Verification items for this drawing (mm, ordinates from the low corner). A direction names the side the tool comes from. Round coordinates to 2 decimals unless told otherwise and drop trailing zeros. Loops run counter-clockwise (first coordinate to the right, second up) from the corner with the lowest first, then second, coordinate; pieces in that order, holes last. Notation, with made-up numbers: M 24,18 L 58,18 A21 cw 58,56 Z; hole C 18,56.25 d3. An arc over 180 degrees is marked long. One line per item, written item: value.
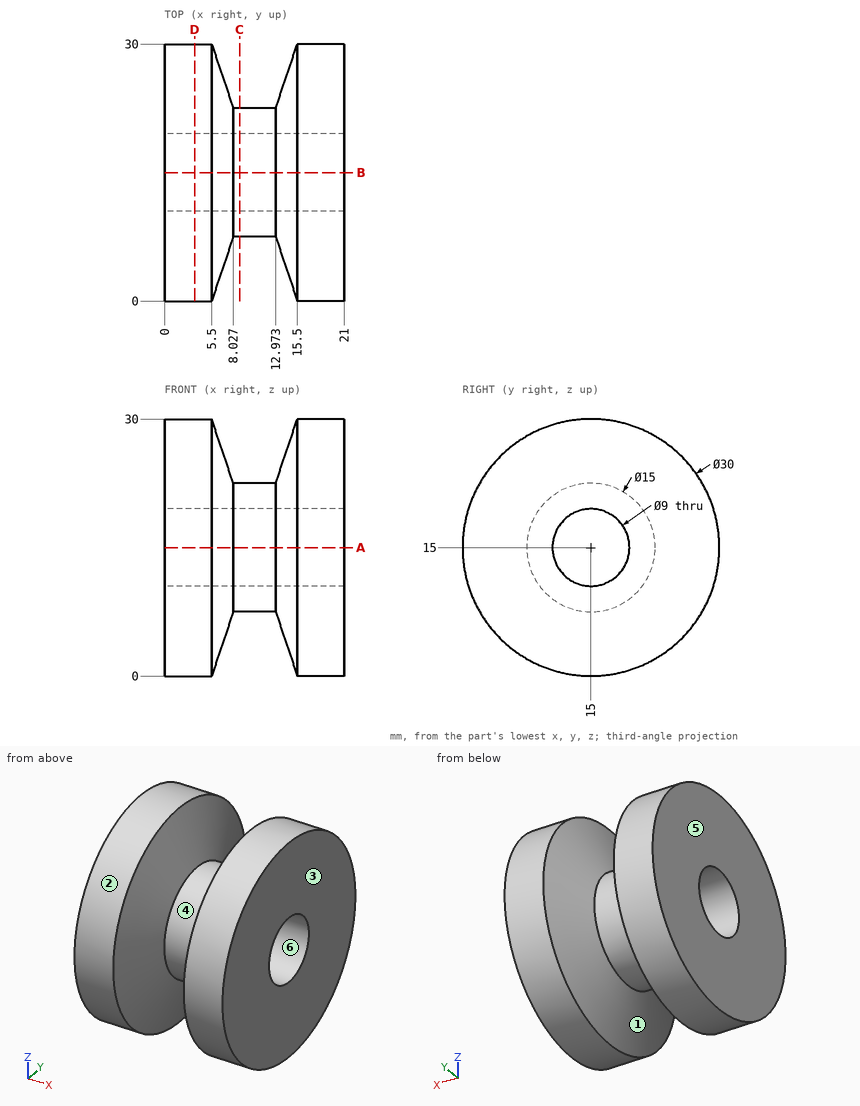
(1) Sectioned sample at D-D on x = 3.5. Enter the section's corners in (y, z).
Completed:
outline: C 15,15 d30; hole C 15,15 d9
(2) Tool access check on the marked faces 1 and 2. Record the directions out of +Z, -Z, +X, -X, +Y, -Y that give a thin tool (end or side, any length) a straight path to the whole face; none if there is none.
Completed:
face 1: none
face 2: +X, -X
(3) Thickness scan on L1, parallel to Z at x = 10, y = 15; L2, parallel to Z at x = 5.25, y = 15; L3, parallel to X at y = 10.75, z = 23.25. Record the ranges inside material, lowest first. Write a range as from..to.
Completed:
L1: z = 7.5..10.5, 19.5..22.5
L2: z = 0..10.5, 19.5..30
L3: x = 0..7.43, 13.57..21
(4) Sectioned sample at C-C on x = 8.75. Enter the section's corners in (y, z).
Completed:
outline: C 15,15 d15; hole C 15,15 d9
(5) Mould release check, pull along X, two halves, no side actions. Record for the marked faces 3, 4, 5 and 6: +X half, -X half, draft (parallel to the pull), parting line (faces both ways), or undercut.
Completed:
face 3: +X half
face 4: undercut
face 5: -X half
face 6: draft
(6) Sectioned sample at A-A on z = 15. Enter the section's corners in (x, y), and give its area (3 significant figures).
Completed:
outline: M 0,0 L 5.5,0 L 8.03,7.5 L 12.97,7.5 L 15.5,0 L 21,0 L 21,10.5 L 0,10.5 Z; M 0,19.5 L 21,19.5 L 21,30 L 15.5,30 L 12.97,22.5 L 8.03,22.5 L 5.5,30 L 0,30 Z
area: 329 mm^2
(7) Depth check by flat-ended pin: pin 1 Ø6 at (x, y) = (17.5, 5.5) entering from +Z; pin 2 Ø5.5 at (y, z) = (15, 15) entering from -X; pin 3 Ø10 at (x, z) = (2.5, 8.5) entering from -Y (3 decimals). Enter the tip coordinate at first touch or a pass-through.
Completed:
pin 1: stops at z = 28.52
pin 2: passes through
pin 3: stops at y = 0.075
